Input: part model. Units: mm. Frame: model coordinates. A direction names the side the tool comes from. Coordinates: 2 decimals unless noted, no trailing zeros. Loops run counter-clockwise (first coordinate to the right, second up) from the corner with the lowest first, then second, coordinate; pieces in that order, holes last. Notation, with made-up numbers: (86.25, 28) - (122.25, 28) arc R31 cw to (122.25, 67) - close; hole circle Ø6 at (-37.75, -16). An arc over 180 degrees is marked (long way). Use one line per item in the form item = value.
from build123d import *

# Parameters (mm, degrees)
F1_DEPTH = 25
F3_D     = 10.8
F4_R     = 5


with BuildPart() as f1:
    # F0 (on Front) → F1 (new body, symmetric)
    with BuildSketch(Plane.XZ):
        Polygon((-25.943926, 37.934126), (-35.943926, 37.934126), (-35.943926, -22.065874), (14.056074, -22.065874), (14.056074, -10.065874), (-25.943926, -10.065874), align=None)
    extrude(amount=F1_DEPTH, both=True)

    # F3 (through all)
    with Locations(Plane.YZ.offset(-25.943926)):
        with Locations((0, 24.934126)):
            Hole(F3_D / 2)

    # F4
    f4_edges = [f1.edges().sort_by_distance(p)[0] for p in [
        (-30.943926, -25, 37.934126),
        (-30.943926, 25, 37.934126),
        (14.056074, -25, -16.065874),
        (14.056074, 25, -16.065874),
        (-35.943926, 0, -22.065874),
        (-25.943926, 0, -10.065874),
    ]]
    fillet(f4_edges, radius=F4_R)


solid = f1.part
Q1. Cut plane A-A, the plane y = 0. Return loops of the section in (x, z), then the cut area to 3 significant figures.
Check values:
outline = (-35.94, -17.07) arc R5 ccw to (-30.94, -22.07) - (14.06, -22.07) - (14.06, -10.07) - (-20.94, -10.07) arc R5 cw to (-25.94, -5.07) - (-25.94, 19.53) - (-35.94, 19.53) - close; (-35.94, 30.33) - (-25.94, 30.33) - (-25.94, 37.93) - (-35.94, 37.93) - close
area = 972 mm²
Q2. Ray query, line 1 along Z through (x, y) = (-30.5, 0); line 2 along X through (y, z) = (-22.5, 19.5); line 3 along Z through (x, y) = (4.5, 16). Return the intervals inside material, ascending. Write a range as [from, to].
Check values:
line_1 = [-22.07, 19.53], [30.33, 37.93]
line_2 = [-35.94, -25.94]
line_3 = [-22.07, -10.07]
Q3. Cut plane D-D, the plane x = -4.5. Return loops of the section in (y, z).
Check values:
outline = (-25, -22.07) - (25, -22.07) - (25, -10.07) - (-25, -10.07) - close
Q4. Set-up query: faces 1 (the flat face through (-9, 0, -22.066)), 2 (the flat face through (-3, 0, -10.066)). Return all of +Z, -Z, +X, -X, +Y, -Y with unobstructed straight access to the full face (end or side cutting, diameter ignored); none if empty.
Check values:
face_1 = -Z, +X, -X, +Y, -Y
face_2 = +Z, +X, +Y, -Y
Q5. Cut plane C-C, the plane z = 7.5. Return loops of the section in (x, y), then the cut area to 3 significant figures.
Check values:
outline = (-35.94, -25) - (-25.94, -25) - (-25.94, 25) - (-35.94, 25) - close
area = 500 mm²
Q6. Cut plane B-B, the plane y = 14. Return loops of the section in (x, z), then the cut area to 3 significant figures.
Check values:
outline = (-35.94, -17.07) arc R5 ccw to (-30.94, -22.07) - (14.06, -22.07) - (14.06, -10.07) - (-20.94, -10.07) arc R5 cw to (-25.94, -5.07) - (-25.94, 37.93) - (-35.94, 37.93) - close
area = 1,080 mm²
Q7. Pull-direction query (Z, two-part tool) for faces 3 (the flat face through (-31, 0, 37.934)), 4 (the flat face through (-25.944, 0, 16)), 5 (the cylindrical face through (-31.01, 0.7, 30.29)); classes: pulls with the +Z half, pulls with the -Z half, needs draft (parallel to the pull), parting line crosses it, or undercut.
Check values:
face_3 = pulls with the +Z half
face_4 = needs draft
face_5 = undercut
Q8. First-contact query: P1, Ø8, axis at y = 17, z = 22.5, coming from the +X side; P2, Ø6.5, axis at y = 0, z = 24.93, coming from the +X side; P3, Ø10, axis at x = 2, y = 9.5, coming from the +Z side. Flat tips, straight axial feed; report the tip coordinate or a pass-through.
Check values:
P1 = -25.94
P2 = through
P3 = -10.07
